Here's how the part is built. I have some questions about the finished solid (model axes, mm). A direction names the side the tool comes from. Round coordinates to 2 decimals unless told otherwise and drop trailing zeros. Loops run counter-clockwise (first coordinate to the right, second up) from the corner with the lowest first, then second, coordinate; pieces in that order, holes last. Notation, with made-up numbers: (16.5, 14) - (24.5, 14) arc R9 cw to (24.5, 18) - close; hole circle Ø6 at (54, 33.5). An arc over 180 degrees is marked (long way). Answer as a JSON object with one key per item and string values. Group by question number.
1) I want a section at B-B, the plane y = -17.5. Please give me the cut outline in (x, z).
2) Will these pins go through, and if not, where does the flat tip stop? P1, Ø6, axis at x = -179, z = 21, coming from the -Y side; P2, Ø5, axis at x = -158, z = 6.5, coming from the -Y side; P3, Ø1.1, axis at x = -159, y = -8.5, coming from the +Z side; P4, Ø12, axis at x = -31, z = -8, coming from the -Y side.
3) Which directions (+Z, -Z, +X, -X, +Y, -Y) give clear straight access to the entire face, cutting with the end or side of a thin tool? Please do faces 1 (the face through (9.299, -53, 13)), 2 (the face through (-156, -13.159, 6)).
4) If I drill on line 1 along X through (y, z) = (-15.5, 7); line 2 along Y through (x, z) = (-57.5, 9.5); line 3 along X through (y, z) = (-42.5, 3), over which ranges is the centre line in solid material (lowest first)? Write a range as [from, to].
5) If we mould it in two halves opening along Y, with no side actions, what happens to faces 3 (the face through (-187, -3.159, 12)), 4 (the face through (-211.7, -0.6, 10.5)), 5 (the face through (-208.701, -1, 12)), 6 (the face through (-50, -6, 0))? For each: pulls with the +Y half, pulls with the -Y half, needs draft (parallel to the pull), parting line crosses it, or undercut.
6) I want a section at A-A, the plane x = -38.5. Please give me the cut outline in (y, z).
from build123d import *

# Parameters (mm, degrees)
ESQUISSE1_W             = 220
ESQUISSE1_H             = 10
ESQUISSE1_W_2           = 10
ESQUISSE1_H_2           = 70
BOSS_EXTRU_1_DEPTH      = 25
BOSS_EXTRU_2_DEPTH      = 12.5
ESQUISSE3_R             = 20
ESQUISSE3_R_2           = 15
BOSS_EXTRU_3_DEPTH      = 10
ENL_V_MAT_EXTRU_1_DEPTH = 227.418066155
ESQUISSE5_W             = 10
ESQUISSE5_H             = 5
ENL_V_MAT_EXTRU_2_DEPTH = 60
ESQUISSE6_R             = 20
BOSS_EXTRU_4_DEPTH      = 4
ESQUISSE8_R             = 2
ENL_V_MAT_EXTRU_4_DEPTH = 6
ESQUISSE10_W            = 5
ESQUISSE10_H            = 10
BOSS_EXTRU_5_DEPTH      = 10
BOSS_EXTRU_6_DEPTH      = 12
BOSS_EXTRU_8_START      = 10
ESQUISSE12_R            = 15
ESQUISSE12_R_2          = 11
BOSS_EXTRU_8_DEPTH      = 10
ENL_V_MAT_EXTRU_5_DEPTH = 20
CONG_1_R                = 2
BOSS_EXTRU_9_START      = 3
ESQUISSE14_R            = 11
BOSS_EXTRU_9_DEPTH      = 3
CONG_2_R                = 5
ESQUISSE16_W            = 5.5
ESQUISSE16_H            = 15
BOSS_EXTRU_10_DEPTH     = 1
ESQUISSE18_W            = 10.448813292
ESQUISSE18_H            = 10
ENL_V_MAT_EXTRU_8_DEPTH = 6
ESQUISSE19_W            = 5
ESQUISSE19_H            = 14.911099914
BOSS_EXTRU_11_DEPTH     = 25


with BuildPart() as part:
    # Esquisse1 → Boss.-Extru.1 (new body)
    with BuildSketch(Plane.XY):
        with Locations((-104.701133521, -3.159392789)):
            Rectangle(ESQUISSE1_W, ESQUISSE1_H)
        with Locations((0.298866479, -43.159392789)):
            Rectangle(ESQUISSE1_W_2, ESQUISSE1_H_2)
    extrude(amount=BOSS_EXTRU_1_DEPTH)

    # Esquisse2 → Boss.-Extru.2 (add, symmetric)
    with BuildSketch(Plane.XY.offset(12.5)):
        Polygon((-160.701133521, 5.840607211), (-162.701133521, 1.840607211), (-158.701133521, 1.840607211), align=None)
        Polygon((-164.701133521, 5.840607211), (-166.701133521, 1.840607211), (-162.701133521, 1.840607211), align=None)
        Polygon((-168.701133521, 5.840607211), (-170.701133521, 1.840607211), (-166.701133521, 1.840607211), align=None)
        Polygon((-172.701133521, 5.840607211), (-174.701133521, 1.840607211), (-170.701133521, 1.840607211), align=None)
        Polygon((-176.701133521, 5.840607211), (-178.701133521, 1.840607211), (-174.701133521, 1.840607211), align=None)
        Polygon((-180.701133521, 5.840607211), (-182.701133521, 1.840607211), (-178.701133521, 1.840607211), align=None)
        Polygon((-184.701133521, 5.840607211), (-186.701133521, 1.840607211), (-182.701133521, 1.840607211), align=None)
        Polygon((-188.701133521, 5.840607211), (-190.701133521, 1.840607211), (-186.701133521, 1.840607211), align=None)
        Polygon((-192.701133521, 5.840607211), (-194.701133521, 1.840607211), (-190.701133521, 1.840607211), align=None)
        Polygon((-196.701133521, 5.840607211), (-198.701133521, 1.840607211), (-194.701133521, 1.840607211), align=None)
        Polygon((-200.701133521, 5.840607211), (-202.701133521, 1.840607211), (-198.701133521, 1.840607211), align=None)
        Polygon((-204.701133521, 5.840607211), (-206.701133521, 1.840607211), (-202.701133521, 1.840607211), align=None)
        Polygon((-208.701133521, 5.840607211), (-210.701133521, 1.840607211), (-206.701133521, 1.840607211), align=None)
        Polygon((-212.701133521, 5.840607211), (-214.701133521, 1.840607211), (-210.701133521, 1.840607211), align=None)
    extrude(amount=BOSS_EXTRU_2_DEPTH, both=True)

    # Esquisse3 → Boss.-Extru.3 (add)
    with BuildSketch(Plane.ZY.offset(4.701133521)):
        with Locations((12.5, -58.159392789)):
            Circle(ESQUISSE3_R)
        with Locations((12.5, -58.159392789)):
            Circle(ESQUISSE3_R_2, mode=Mode.SUBTRACT)
    extrude(amount=-BOSS_EXTRU_3_DEPTH)

    # Esquisse4 → Enl_v. mat.-Extru.1 (cut, through all)
    with BuildSketch(Plane.ZY.offset(4.701133521)):
        with BuildLine():
            Line((25, -66.450954765), (25, -49.867830813))
            ThreePointArc((25, -49.867830813), (12.5, -43.159392789), (0, -49.867830813))
            Line((0, -49.867830813), (0, -66.450954765))
            ThreePointArc((0, -66.450954765), (12.5, -73.159392789), (25, -66.450954765))
        make_face()
        with BuildLine():
            Line((25, -78.159392789), (25, -73.771887785))
            ThreePointArc((25, -73.771887785), (19.123824427, -77.03066593), (12.5, -78.159392789))
            Line((12.5, -78.159392789), (25, -78.159392789))
        make_face()
        with BuildLine():
            ThreePointArc((12.5, -78.159392789), (5.876175573, -77.03066593), (0, -73.771887785))
            Line((0, -73.771887785), (0, -78.159392789))
            Line((0, -78.159392789), (12.5, -78.159392789))
        make_face()
    extrude(amount=-ENL_V_MAT_EXTRU_1_DEPTH, mode=Mode.SUBTRACT)

    # Esquisse5 → Enl_v. mat.-Extru.2 (cut)
    with BuildSketch(Plane.ZY.offset(214.701133521)):
        with Locations((12.5, -5.659392789)):
            Rectangle(ESQUISSE5_W, ESQUISSE5_H)
    extrude(amount=-ENL_V_MAT_EXTRU_2_DEPTH, mode=Mode.SUBTRACT)

    # Esquisse6 → Boss.-Extru.4 (add)
    with BuildSketch(Plane(origin=(5.298866479, 0, 0), x_dir=(0, 0, -1), z_dir=(1, 0, 0))):
        with Locations(Location((-12.5, -58.159392789, 0), (0, 0, 51.317812547))):
            Circle(ESQUISSE6_R)
    extrude(amount=BOSS_EXTRU_4_DEPTH)

    # Esquisse8 → Enl_v. mat.-Extru.4 (cut)
    with BuildSketch(Plane.ZY.offset(214.701133521)):
        with Locations((12.5, -0.659392789)):
            Circle(ESQUISSE8_R)
    extrude(amount=-ENL_V_MAT_EXTRU_4_DEPTH, mode=Mode.SUBTRACT)

    # Esquisse10 → Boss.-Extru.5 (add)
    with BuildSketch(Plane.XY.offset(25)):
        with Locations((-156.201133521, -3.159392789)):
            Rectangle(ESQUISSE10_W, ESQUISSE10_H)
    extrude(amount=BOSS_EXTRU_5_DEPTH)

    # Esquisse11 → Boss.-Extru.6 (add)
    with BuildSketch(Plane(origin=(0, 0, 0), x_dir=(-1, 0, 0), z_dir=(0, 0, -1))):
        Polygon((153.701133521, -8.159392789), (153.701133521, -13.159392789), (158.701133521, -13.159392789), (158.701133521, -8.159392789), (158.701133521, 1.840607211), (153.701133521, 1.840607211), align=None)
    extrude(amount=BOSS_EXTRU_6_DEPTH)

    # Esquisse12 → Boss.-Extru.8 (add)
    with BuildSketch(Plane.ZY.offset(-5.298866479).offset(BOSS_EXTRU_8_START)):
        with Locations((12.5, -58.159392789)):
            Circle(ESQUISSE12_R)
        with Locations(Location((12.5, -58.159392789, 0), (0, 0, 270))):
            Circle(ESQUISSE12_R_2, mode=Mode.SUBTRACT)
    extrude(amount=-BOSS_EXTRU_8_DEPTH)

    # Esquisse13 → Enl_v. mat.-Extru.5 (cut)
    with BuildSketch(Plane.ZY.offset(4.701133521)):
        with BuildLine():
            Line((0, -58.159392789), (0, -42.546897793))
            ThreePointArc((0, -42.546897793), (3.839745962, -76.187149167), (32.5, -58.159392789))
            ThreePointArc((32.5, -58.159392789), (30.527756377, -49.499138752), (25, -42.546897793))
            Line((25, -42.546897793), (25, -58.159392789))
            ThreePointArc((25, -58.159392789), (12.5, -70.659392789), (0, -58.159392789))
        make_face()
    extrude(amount=-ENL_V_MAT_EXTRU_5_DEPTH, mode=Mode.SUBTRACT)

    # Cong_1
    # the kernel refuses this fillet: 2 mm, written as the material it takes off along each edge
    with BuildSketch(Plane(origin=(9.298866479, -58.159392789, 12.5), x_dir=(0, 0.601670275435169, -0.7987445647125042), z_dir=(0, -0.7987445647125042, -0.601670275435169))) as cong_1_piece_1:
        with BuildLine():
            CenterArc((20 - CONG_1_R, -CONG_1_R), CONG_1_R, 0, 90)
            Line((20, -CONG_1_R), (20, 0))
            Line((20, 0), (20 - CONG_1_R, 0))
        make_face()
    revolve(axis=Axis((9.298866479, -58.159392789, 12.5), (1, 0, 0)), revolution_arc=106.02076759, mode=Mode.SUBTRACT)
    with BuildSketch(Plane(origin=(9.298866479, -37.546897793, 0), x_dir=(-1, 0, 0), z_dir=(0, -1, 0))) as cong_1_piece_2:
        with BuildLine():
            CenterArc((CONG_1_R, -CONG_1_R), CONG_1_R, 90, 90)
            Line((0, -CONG_1_R), (0, 0))
            Line((0, 0), (CONG_1_R, 0))
        make_face()
    extrude(amount=20.612494996, mode=Mode.SUBTRACT)
    with BuildSketch(Plane(origin=(9.298866479, -58.159392789, 12.5), x_dir=(0, 0, -1), z_dir=(0, 1, 0))) as cong_1_piece_3:
        with BuildLine():
            CenterArc((12.5 - CONG_1_R, CONG_1_R), CONG_1_R, 270, 90)
            Line((12.5 - CONG_1_R, 0), (12.5, 0))
            Line((12.5, 0), (12.5, CONG_1_R))
        make_face()
    revolve(axis=Axis((9.298866479, -58.159392789, 12.5), (-1, 0, 0)), revolution_arc=180, mode=Mode.SUBTRACT)
    with BuildSketch(Plane(origin=(9.298866479, -58.159392789, 25), x_dir=(0, 0, -1), z_dir=(0, 1, 0))) as cong_1_piece_4:
        with BuildLine():
            CenterArc((CONG_1_R, CONG_1_R), CONG_1_R, 180, 90)
            Line((0, CONG_1_R), (0, 0))
            Line((0, 0), (CONG_1_R, 0))
        make_face()
    extrude(amount=20.612494996, mode=Mode.SUBTRACT)

    # Esquisse14 → Boss.-Extru.9 (add)
    with BuildSketch(Plane.ZY.offset(-5.298866479).offset(BOSS_EXTRU_9_START)):
        with Locations(Location((12.5, -58.159392789, 0), (0, 0, 270))):
            Circle(ESQUISSE14_R)
    extrude(amount=-BOSS_EXTRU_9_DEPTH)

    # Cong_2
    cong_2_edges = [part.edges().sort_by_distance(p)[0] for p in [
        (-4.701133521, -8.159392789, 12.5),
        (5.298866479, 1.840607211, 12.5),
    ]]
    fillet(cong_2_edges, radius=CONG_2_R)

    # Esquisse16 → Boss.-Extru.10 (add)
    with BuildSketch(Plane.ZY.offset(158.701133521)):
        with Locations((-9.25, -5.659392789)):
            Rectangle(ESQUISSE16_W, ESQUISSE16_H)
    extrude(amount=BOSS_EXTRU_10_DEPTH)

    # Esquisse18 → Enl_v. mat.-Extru.8 (cut)
    with BuildSketch(Plane.ZY.offset(158.701133521)):
        with Locations((30.224406646, -3.159392789)):
            Rectangle(ESQUISSE18_W, ESQUISSE18_H)
    extrude(amount=-ENL_V_MAT_EXTRU_8_DEPTH, mode=Mode.SUBTRACT)

    # Esquisse19 → Boss.-Extru.11 (add)
    with BuildSketch(Plane.XY):
        with Locations((-156.201133521, -5.703842832)):
            Rectangle(ESQUISSE19_W, ESQUISSE19_H)
    extrude(amount=BOSS_EXTRU_11_DEPTH)


solid = part.part
Outcome:
{
 "1": {"outline": "(-4.7, 0) - (5.3, 0) - (5.3, 25) - (-4.7, 25) - close"},
 "2": {"P1": "y = -8.16", "P2": "y = -13.16", "P3": "z = 25", "P4": "through"},
 "3": {"face 1": "+Z, -Z, +X, +Y, -Y", "face 2": "+Z, -Z, -X, -Y"},
 "4": {"line 1": "[-4.7, 5.3]", "line 2": "[-8.16, 1.84]", "line 3": "[-4.7, 9.27]"},
 "5": {"face 3": "pulls with the -Y half", "face 4": "undercut", "face 5": "undercut", "face 6": "needs draft"},
 "6": {"outline": "(-8.16, 0) - (1.84, 0) - (1.84, 25) - (-8.16, 25) - close"}
}
